Part model, mm, in its own coordinate system. Face numbers are marked on the shaded views. Coordinates: 2 decimals unless noted, no trailing zeros. Write each loop counter-clockwise with the first axis right and the second up, starting at its lowest first coordinate (ties: lowest second). Pieces come first, ordered by that corner, then holes. Notation, with made-up numbers: (19.25, 0) - (78.25, 0) arc R24 cw to (78.25, 23) - close; hole circle Ø1 at (27.5, 64). An arc over 180 degrees is marked (long way). Use one line per item in the form item = value. Start each with the question number.
Solid Edge part; units mm, degrees
sketch "Sketch1" plane through (0, 0, 0) normal (0, 0, 1) x (1, 0, 0)
  circle A0 centre (0, 0) radius 15
extrude "Protrusion1" add sketch "Sketch1" along normal mid plane 7
sketch "Sketch2" plane through (0, 0, 3.5) normal (0, 0, 1) x (1, 0, 0)
  circle A0 centre (0, 0) radius 11
extrude "ExtrudedCutout_2" cut sketch "Sketch2" against normal blind 28.5
sketch "Sketch3" plane through (0, 0, -3.5) normal (0, 0, -1) x (1, 0, 0)
  circle A0 centre (0, 0) radius 15
extrude "ExtrudedProtrusion_2" add sketch "Sketch3" along normal blind 1
sketch "Sketch4" plane through (0, 0, -4.5) normal (0, 0, -1) x (1, 0, 0)
  circle A0 centre (0, 0) radius 4.5
extrude "ExtrudedCutout_3" cut sketch "Sketch4" against normal blind 57
sketch "Sketch5" plane through (0, 0, 3.5) normal (0, 0, 1) x (1, 0, 0)
  circle A0 centre (0, 0) radius 15
extrude "ExtrudedProtrusion_3" add sketch "Sketch5" along normal blind 4
sketch "Sketch6" plane through (0, 0, 7.5) normal (0, 0, 1) x (1, 0, 0)
  circle A0 centre (0, 0) radius 11
extrude "ExtrudedCutout_4" cut sketch "Sketch6" against normal blind 4
chamfer "Chamfer_1" distance 4 angle 45 1 edges at (-15, 0, 7.5)
sketch "Sketch7" plane through (0, 0, -4.5) normal (0, 0, -1) x (-1, 0, 0)
  circle A0 centre (0, 0) radius 15
extrude "ExtrudedProtrusion_5" add sketch "Sketch7" along normal blind 4
sketch "Sketch8" plane through (0, 0, -8.5) normal (0, 0, -1) x (-1, 0, 0)
  circle A0 centre (0, 0) radius 4.5
extrude "ExtrudedCutout_6" cut sketch "Sketch8" against normal blind 47.5
chamfer "Chamfer_3" distance 4 angle 45 1 edges at (15, 0, -8.5)
sketch "Sketch9" plane through (0, 0, -8.5) normal (0, 0, -1) x (-1, 0, 0)
  circle A0 centre (0, 0) radius 4.5
extrude "Protrusion2" add sketch "Sketch9" against normal up to vertex (5 mm away)
sketch "Sketch10" plane through (0, 0, -3.5) normal (0, 0, 1) x (0, 1, 0)
  circle A0 centre (0, 0) radius 3.5
extrude "ExtrudedProtrusion_7" add sketch "Sketch10" along normal blind 7
sketch "Sketch11" plane through (0, 0, 3.5) normal (0, 0, 1) x (0, 1, 0)
  circle A0 centre (0, 0) radius 2.5
extrude "ExtrudedCutout_7" cut sketch "Sketch11" against normal blind 266
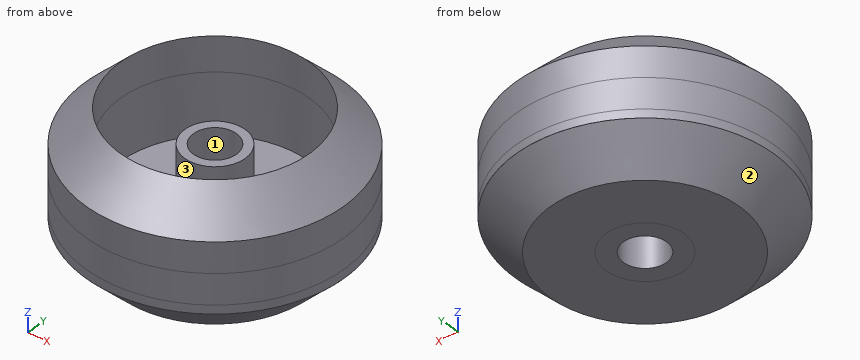
Q1. Slice it at C-C (z = 0.75). List the corners of the cut face in (x, y).
Q2. Pin check, flat tips, straight feed: P1, Ø1, axis at x = -8, z = 5, coming from the -Y side; P2, Ø1, axis at y = 12, z = -2, coming from the -X side; P3, Ø7, axis at x = -2, y = -0.5, coming from the +Z side. Stop position of each tip, or through.
Q3. Drill centre lines: probe 1 along Y at (x, z) = (0, -1.75); probe 2 along X at (y, z) = (-1.75, 1); probe 3 along X at (y, z) = (0, -4.25). Where is each one in solid material? Low to high.
Q4. Slice it at D-D (z = 5). List the corners of the cut face in (x, y).
Q5. Mould opens along X. For the marked faces 1, 2 and 3 say: released by +X, released by -X, zero draft, split by the parting line, or undercut.
Solution:
q1.outline = circle Ø30 at (0, 0); circle Ø7 at (0, 0); hole circle Ø22 at (0, 0); hole circle Ø5 at (0, 0)
q2.P1 = -11.58
q2.P2 = -9.63
q2.P3 = 3.5
q3.probe_1 = -15 to -11, -3.5 to -2.5, 2.5 to 3.5, 11 to 15
q3.probe_2 = -14.9 to -10.86, -3.03 to -1.79, 1.79 to 3.03, 10.86 to 14.9
q3.probe_3 = -15 to -2.5, 2.5 to 15
q4.outline = circle Ø27 at (0, 0); hole circle Ø22 at (0, 0)
q5.face_1 = undercut
q5.face_2 = split by the parting line
q5.face_3 = undercut
